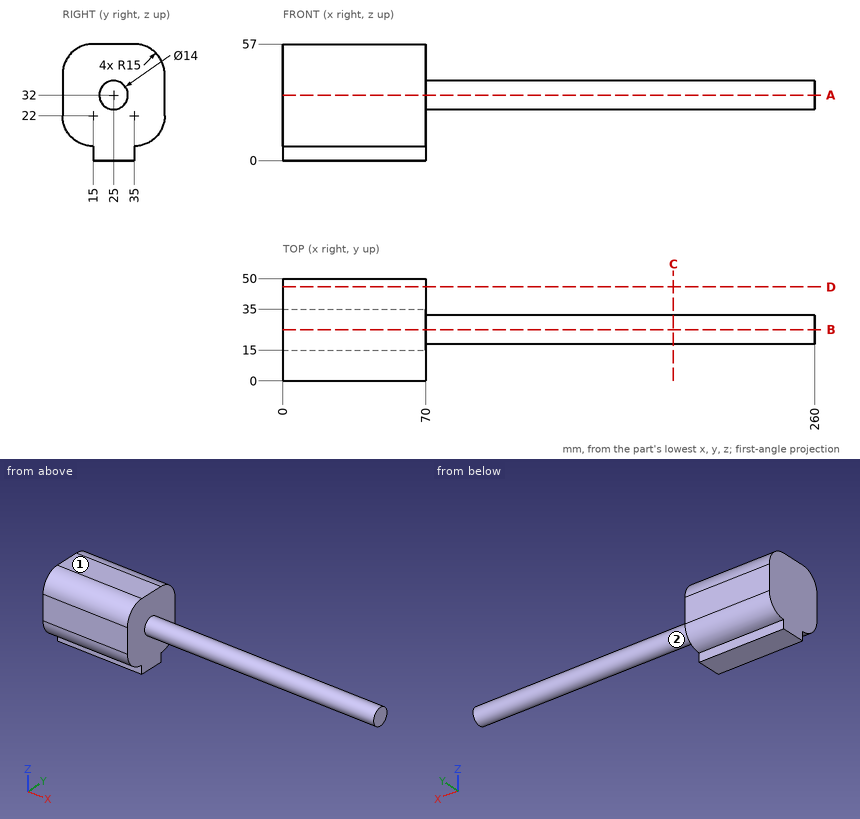
Check sheet for the drawn part. Datum: minimum x, y, z corner. Units: mm. A direction names the side the tool comes from. Give positions to 0.01 mm unless a question says otherwise; leave off trailing zeros. Order: outer loops, then holes, each group sorted by start corner. A loop starts at its lowest first (then second) coordinate and runs counter-clockwise, first axis right, second up.
1. Access from +Z, -Z, +X, -X, +Y, -Y to the whole of each face (thin tool, end or side, straight path). Record for the marked faces 1 and 2.
Completed:
face 1: +Z, +X, -X, +Y, -Y
face 2: +X
2. Depth check by flat-ended pin: pin 1 (8 mm diameter, centred on y = 41, z = 41.5, fed in from +X); pin 2 (2 mm diameter, centred on x = 158, z = 28, fed in from +Y); pin 3 (2 mm diameter, centred on x = 159, y = 19.5, fed in from -Z). Enter the tip coordinate at first touch or a pass-through.
Completed:
pin 1: stops at x = 70
pin 2: stops at y = 31.32
pin 3: stops at z = 26.64
3. Scan lines: line 1 (X direction, y = 46, z = 28.5); line 2 (Z direction, x = 65, y = 35.5); line 3 (Z direction, x = 25.5, y = 47). Record each from-to range of solid material in increasing order.
Completed:
line 1: x = 0 to 70
line 2: z = 7.01 to 56.99
line 3: z = 13 to 51
4. Sectioned sample at C-C (x = 191). Record the boundary of the cut face in (y, z).
Completed:
outline: circle Ø14 at (25, 32)
5. Sectioned sample at A-A (z = 32). Record the boundary of the cut face in (x, y), then the cut area to 3 significant figures.
Completed:
outline: (0, 0) - (70, 0) - (70, 18) - (260, 18) - (260, 32) - (70, 32) - (70, 50) - (0, 50) - close
area: 6,160 mm2
6. Sectioned sample at D-D (y = 46). Record the boundary of the cut face in (x, z), then the cut area to 3 significant figures.
Completed:
outline: (0, 11.8) - (70, 11.8) - (70, 52.2) - (0, 52.2) - close
area: 2,830 mm2
7. Sectioned sample at B-B (y = 25). Record the boundary of the cut face in (x, z), then the cut area to 3 significant figures.
Completed:
outline: (0, 0) - (70, 0) - (70, 25) - (260, 25) - (260, 39) - (70, 39) - (70, 57) - (0, 57) - close
area: 6,650 mm2
